from build123d import *

# Parameters (mm, degrees)
SKETCH1_R           = 3.81
SKETCH1_R_2         = 3.31
BOSS_EXTRUDE1_DEPTH = 2.4
BOSS_EXTRUDE2_DEPTH = 6.1
SKETCH4_R           = 3.1
BOSS_EXTRUDE3_DEPTH = 1.4
SKETCH5_W           = 6.5
SKETCH5_H           = 6.7
BOSS_EXTRUDE4_DEPTH = 7
SKETCH6_R           = 2.5
SKETCH6_R_2         = 2.45
CUT_EXTRUDE1_DEPTH  = 7
CUT_EXTRUDE2_DEPTH  = 0.5
SKETCH8_R           = 4.075
BOSS_EXTRUDE5_DEPTH = 1.4
SKETCH9_R           = 3.6
BOSS_EXTRUDE6_DEPTH = 2.3
SKETCH10_R          = 4.125
BOSS_EXTRUDE7_DEPTH = 3.25


with BuildPart() as part:
    # Sketch1 → Boss-Extrude1 (new body)
    with BuildSketch(Plane.XY):
        Circle(SKETCH1_R)
        Circle(SKETCH1_R_2, mode=Mode.SUBTRACT)
    extrude(amount=BOSS_EXTRUDE1_DEPTH)

    # Sketch2 → Boss-Extrude2 (add)
    with BuildSketch(Plane(origin=(0, 0, 0), x_dir=(-1, 0, 0), z_dir=(0, 0, -1))):
        Polygon((2.309401077, -4), (4.618802154, 0), (2.309401077, 4), (-2.309401077, 4), (-4.618802154, 0), (-2.309401077, -4), align=None)
    extrude(amount=BOSS_EXTRUDE2_DEPTH)

    # Sketch3 → Cut-Revolve1 (revolve, cut)
    with BuildSketch(Plane(origin=(0, 0, 0), x_dir=(1, 0, 0), z_dir=(0, 1, 0))):
        with BuildLine():
            Line((-4.618802154, 5.6), (-4.618802154, 6.1))
            Line((-4.618802154, 6.1), (-4.118802154, 6.1))
            ThreePointArc((-4.118802154, 6.1), (-4.472355544, 5.953553391), (-4.618802154, 5.6))
        make_face()
        with BuildLine():
            Line((-4.618802154, 0), (-4.118802154, 0))
            ThreePointArc((-4.118802154, 0), (-4.472355544, 0.146446609), (-4.618802154, 0.5))
            Line((-4.618802154, 0.5), (-4.618802154, 0))
        make_face()
    revolve(axis=Axis((0, 0, 0), (0, 0, -1)), mode=Mode.SUBTRACT)

    # Sketch4 → Boss-Extrude3 (add)
    with BuildSketch(Plane(origin=(0, 0, -6.1), x_dir=(-1, 0, 0), z_dir=(0, 0, -1))):
        Circle(SKETCH4_R)
    extrude(amount=BOSS_EXTRUDE3_DEPTH)

    # Sketch5 → Boss-Extrude4 (add)
    with BuildSketch(Plane(origin=(0, 0, -7.5), x_dir=(-1, 0, 0), z_dir=(0, 0, -1))):
        Rectangle(SKETCH5_W, SKETCH5_H)
    extrude(amount=BOSS_EXTRUDE4_DEPTH)

    # Sketch6 → Cut-Extrude1 (cut)
    with BuildSketch(Plane(origin=(0, 0, -14.5), x_dir=(-1, 0, 0), z_dir=(0, 0, -1))):
        Circle(SKETCH6_R)
        Circle(SKETCH6_R_2, mode=Mode.SUBTRACT)
    extrude(amount=-CUT_EXTRUDE1_DEPTH, mode=Mode.SUBTRACT)

    # Sketch7 → Cut-Extrude2 (cut)
    with BuildSketch(Plane(origin=(0, 0, -14.5), x_dir=(-1, 0, 0), z_dir=(0, 0, -1))):
        with BuildLine():
            Line((1.462150124, 2.027835549), (-2.027835549, -1.462150124))
            ThreePointArc((-2.027835549, -1.462150124), (-1.767766953, -1.767766953), (-1.462150124, -2.027835549))
            Line((-1.462150124, -2.027835549), (2.027835549, 1.462150124))
            ThreePointArc((2.027835549, 1.462150124), (1.767766953, 1.767766953), (1.462150124, 2.027835549))
        make_face()
    extrude(amount=-CUT_EXTRUDE2_DEPTH, mode=Mode.SUBTRACT)

    # Sketch8 → Boss-Extrude5 (add)
    with BuildSketch(Plane(origin=(0, 3.35, 0), x_dir=(1, 0, 0), z_dir=(0, 1, 0))):
        with Locations(Location((0, 11, 0), (0, 0, 59.192817964))):
            Circle(SKETCH8_R)
    extrude(amount=BOSS_EXTRUDE5_DEPTH)

    # Sketch9 → Boss-Extrude6 (add)
    with BuildSketch(Plane(origin=(0, 4.75, 0), x_dir=(1, 0, 0), z_dir=(0, 1, 0))):
        with Locations(Location((0, 11, 0), (0, 0, 270))):
            Circle(SKETCH9_R)
    extrude(amount=BOSS_EXTRUDE6_DEPTH)

    # Sketch10 → Boss-Extrude7 (add)
    with BuildSketch(Plane(origin=(0, 7.05, 0), x_dir=(1, 0, 0), z_dir=(0, 1, 0))):
        with Locations(Location((0, 11, 0), (0, 0, 90))):
            Circle(SKETCH10_R)
    extrude(amount=BOSS_EXTRUDE7_DEPTH)

    # Sketch11 → Revolve1 (revolve)
    with BuildSketch(Plane(origin=(0, 0, 0), x_dir=(0, 0, -1), z_dir=(1, 0, 0)), mode=Mode.PRIVATE) as revolve1_sk:
        with BuildLine():
            Line((11, 10.3), (5.9, 10.3))
            ThreePointArc((5.9, 10.3), (5.987513668, 17.302187158), (6.25, 24.3))
            ThreePointArc((6.25, 24.3), (6.932343055, 34.067289726), (8, 43.8))
            ThreePointArc((8, 43.8), (9.047437581, 45.593074903), (11, 46.3))
            Line((11, 46.3), (11, 10.3))
        make_face()
    revolve(revolve1_sk.sketch.rotate(Axis((0, 10.3, -11), (0, 1, 0)), 180), axis=Axis((0, 10.3, -11), (0, 1, 0)))


solid = part.part
Check sheet for the modelled part. Datum: model origin and axes. Units: mm. A direction names the side the tool comes from. Round coordinates to 2 decimals unless told otherwise and drop trailing zeros.
(1) Scan lines: probe 1 along Y at (x, z) = (0, 0.75); probe 2 along X at (y, z) = (38.5, -11.5); probe 3 along Y at (x, z) = (2.25, -3). Record each from-to range of solid material in increasing order.
(2) Go/stop test with flat-tipped pins: P1, Ø7.5, axis at y = -0.5, z = -12.5, coming from the -X side; P2, Ø0.7, axis at x = 3.5, z = -10, coming from the -Y side; P3, Ø8, axis at y = 22.5, z = -3, coming from the +X side. Record where each tip stops, or that it passes through.
(3) Access from +Z, -Z, +X, -X, +Y, -Y to the whole of each face (thin tool, end or side, straight path). Record for faces 1 (the flat face through (-3.448, -2.028, -3.007)), 2 (the flat face through (-0.259, -0.307, -14.254)), 3 (the flat face through (0, 0, 0)), 4 (the cylindrical face through (-0.18, 8.65, -6.88)).
(4) Draft check along Y on faces 5 (the flat face through (-1, -1, -14.5)), 6 (the flat face through (3.48, -1.97, -3.01)), 7 (the cylindrical face through (1.081, 5.884, -7.566)). Enter one of: pulls with the +Y half, pulls with the -Y half, needs draft (parallel to the pull), parting line crosses it, or undercut.
(5) Cross-section at A-A, the plane z = -11. State how many separate pieces and enclosed holes the cut face has, and give its area (3 significant figures).
Check sheet entries:
1. probe 1: y = -3.81 to -3.31, 3.31 to 3.81
1. probe 2: x = -3.6 to 3.6
1. probe 3: y = -4 to 4
2. P1: stops at x = -3.25
2. P2: stops at y = -3.35
2. P3: stops at x = 2.72
3. face 1: +Z, -X, -Y
3. face 2: -Z
3. face 3: +Z
3. face 4: none
4. face 5: needs draft
4. face 6: pulls with the -Y half
4. face 7: undercut
5. separate pieces: 2
5. enclosed holes: 1
5. area: 405 mm2
